from build123d import *

# Parameters (mm, degrees)
CROQUIS1_W              = 40
CROQUIS1_H              = 40
SALIENTE_EXTRUIR1_DEPTH = 186
SALIENTE_EXTRUIR2_DEPTH = 40


with BuildPart() as part:
    # Croquis1 → Saliente-Extruir1 (new body)
    with BuildSketch(Plane.XY):
        Rectangle(CROQUIS1_W, CROQUIS1_H)
    extrude(amount=SALIENTE_EXTRUIR1_DEPTH)

    # Croquis4 → Saliente-Extruir2 (add)
    with BuildSketch(Plane(origin=(20, 0, 0), x_dir=(0, 0, -1), z_dir=(1, 0, 0))):
        Polygon((0, -20), (20, 0), (18, 0), (0, -18), align=None)
        Polygon((20, 0), (0, 20), (0, 18), (18, 0), align=None)
        Polygon((-186, 18), (-186, 20), (-206, 0), (-204, 0), align=None)
        Polygon((-204, 0), (-206, 0), (-186, -20), (-186, -18), align=None)
    extrude(amount=-SALIENTE_EXTRUIR2_DEPTH)


solid = part.part
Read the model definition and answer for the solid it produces. Units are mm, in the model's axes. A direction names the side the tool comes from. Round coordinates to 2 decimals unless told otherwise and drop trailing zeros. Write each loop counter-clockwise with the first axis right and the second up, starting at its lowest first coordinate (ties: lowest second). Pieces come first, ordered by that corner, then holes.
1. Given pin 1 Ø8 at (x, y) = (-4.5, 7.5) entering from +Z; pin 2 Ø10 at (x, y) = (3, -9.5) entering from +Z; pin 3 Ø1.5 at (x, y) = (2.5, -11) entering from -Z, each flat-ended and moving along its own axis, determine where each tip first touches the part or whether it passes through.
2. The part is cut by section A-A, the plane z = 188. Determine the outline of the cut face in (x, y).
3. Straight lines are drawn through the part: L1, parallel to Z at x = -5, y = -12; L2, parallel to Z at x = -4.5, y = -3; L3, parallel to Y at x = 17, z = 193. For each, find the intervals that lie inside material, in ascending order.
4. The part is cut by section B-B, the plane y = 5. Determine the outline of the cut face in (x, z), then the cut area to 3 significant figures.
5. The part is cut by section C-C, the plane x = 13.5. Determine the outline of the cut face in (y, z), then the cut area to 3 significant figures.
6. Determine the mould class of faces 3 (the face through (20, 0, 95)), 4 (the face through (0, -10, -10)), 5 (the face through (0, 9, 195)) for opening direction Z: pulls with the +Z half, pulls with the -Z half, needs draft (parallel to the pull), parting line crosses it, or undercut.
7. Which of the six approach directions +Z, -Z, +X, -X, +Y, -Y give full straight-line access (tool end or side, diameter ignored) to faces 1 (the face through (0, -9, -9)), 2 (the face through (0, -20, 92))?
Values:
1. pin 1: stops at z = 202.5
1. pin 2: stops at z = 201.5
1. pin 3: stops at z = -9.75
2. outline: (-20, -18) - (20, -18) - (20, -16) - (-20, -16) - close; (-20, 16) - (20, 16) - (20, 18) - (-20, 18) - close
3. L1: z = -8 to -6, 0 to 186, 192 to 194
3. L2: z = -17 to -15, 0 to 186, 201 to 203
3. L3: y = -13 to -11, 11 to 13
4. outline: (-20, -15) - (20, -15) - (20, -13) - (-20, -13) - close; (-20, 0) - (20, 0) - (20, 186) - (-20, 186) - close; (-20, 199) - (20, 199) - (20, 201) - (-20, 201) - close
4. area: 7,600 mm2
5. outline: (-20, 0) - (0, -20) - (20, 0) - (20, 186) - (0, 206) - (-20, 186) - close; hole (-18, 0) - (0, -18) - (18, 0) - close; hole (-18, 186) - (18, 186) - (0, 204) - close
5. area: 7,590 mm2
6. face 3: needs draft
6. face 4: pulls with the -Z half
6. face 5: undercut
7. face 1: +X, -X
7. face 2: +Z, -Z, +X, -X, -Y
